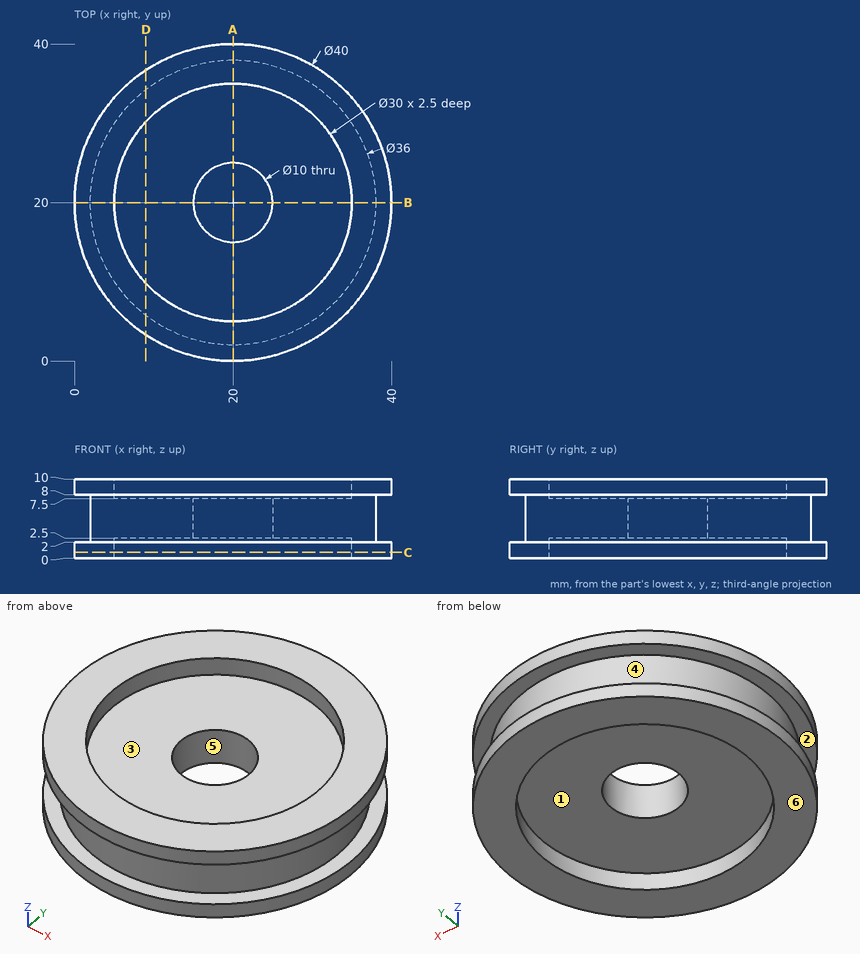
Part print with two shaded views. Sizes in mm from the minimum x, y, z corner. A direction names the side the tool comes from. Give positions to 0.01 mm unless a question says otherwise; leave off trailing zeros. Order: outer loops, then holes, each group sorted by start corner. A loop starts at its lowest first (then second) coordinate and runs counter-clockwise, first axis right, second up. Notation, with made-up numbers: M 66.25,81.25 L 100.25,81.25 A27 ccw 100.25,106.25 Z; hole C 7.5,3.5 d7. An arc over 180 degrees is marked long. Put each result on its own line as item: value.
Item 1: Cut at D-D on x = 9. Write the cut outline in (y, z), then the cut area to 3 significant figures.
Results are:
outline: M 3.3,0 L 9.8,0 L 9.8,2.5 L 30.2,2.5 L 30.2,0 L 36.7,0 L 36.7,2 L 34.25,2 L 34.25,8 L 36.7,8 L 36.7,10 L 30.2,10 L 30.2,7.5 L 9.8,7.5 L 9.8,10 L 3.3,10 L 3.3,8 L 5.75,8 L 5.75,2 L 3.3,2 Z
area: 203 mm2
Item 2: Pull direction X, two halves, no side cores. Call the marked faces 4, 5 and 6: +X half, -X half, draft (parallel to the pull), parting line (faces both ways), or undercut.
Results are:
face 4: parting line
face 5: undercut
face 6: draft
Item 3: Cut at C-C on z = 0.75. Write the cut outline in (x, y), then the cut area to 3 significant figures.
Results are:
outline: C 20,20 d40; hole C 20,20 d30
area: 550 mm2
Item 4: Drop flat-ended pins along their axis: pin 1 Ø2 at (x, z) = (29, 2) entering from -Y; pin 2 Ø3 at (y, z) = (31.5, 1.5) entering from +X; pin 3 Ø5 at (x, z) = (34, 6.5) entering from +Y; pin 4 Ø6 at (x, y) = (20, 20) entering from -Z. Give the stop position or say it passes through.
Results are:
pin 1: y = 1.67
pin 2: x = 37.32
pin 3: y = 36
pin 4: through
Item 5: Wall check: probe 1 along Z at (x, y) = (8, 5.5); probe 2 along X at (y, z) = (20, 1.7); probe 3 along Y at (x, z) = (20, 5.45). Give the ranges that are in metal, low to high.
Results are:
probe 1: 0 to 2, 8 to 10
probe 2: 0 to 5, 35 to 40
probe 3: 2 to 15, 25 to 38
Item 6: Which spindle directions (+Z, -Z, +X, -X, +Y, -Y) get a long thin tool onto all of the face, cutting with end or side? Do the marked faces 1, 2 and 3. Say none if no direction does.
Results are:
face 1: -Z
face 2: none
face 3: +Z
Item 7: Cut at A-A on x = 20. Write the cut outline in (y, z).
Results are:
outline: M 0,0 L 5,0 L 5,2.5 L 15,2.5 L 15,7.5 L 5,7.5 L 5,10 L 0,10 L 0,8 L 2,8 L 2,2 L 0,2 Z; M 25,2.5 L 35,2.5 L 35,0 L 40,0 L 40,2 L 38,2 L 38,8 L 40,8 L 40,10 L 35,10 L 35,7.5 L 25,7.5 Z
